Geometry check sheet. Reference: drawing and pictorial views, mm from the part's lowest x, y, z. A direction names the side the tool comes from. Give positions to 0.01 mm unless a question says otherwise; leave off trailing zeros. Order: outer loops, then holes, each group sorted by start corner. A loop starts at its lowest first (then second) coordinate and runs counter-clockwise, first axis right, second up. Notation, with made-up numbers: (20.5, 64) - (74.5, 64) arc R16 ccw to (74.5, 77) - close; hole circle Ø3 at (35.25, 23). An arc over 180 degrees is marked (long way). Answer as a JSON object with one key per item and string values.
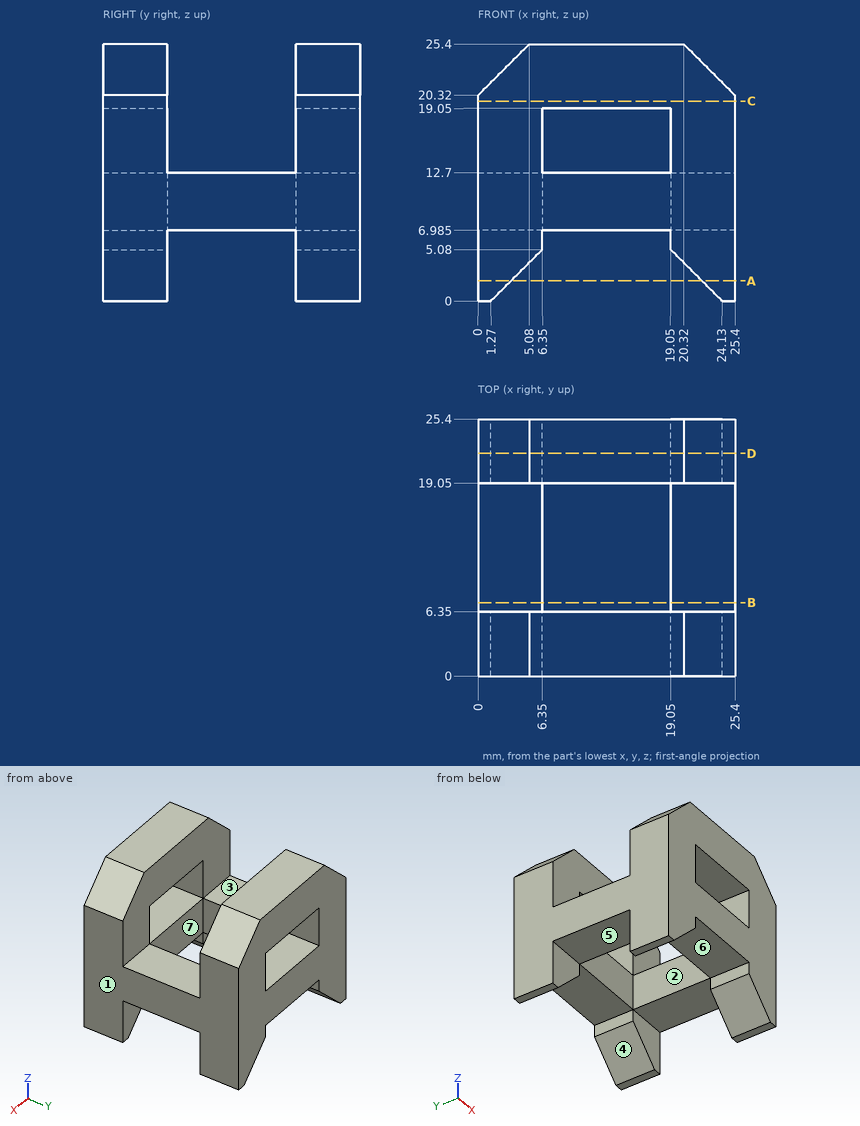
(1) Section check B-B (y = 7.25). Record the cut outline in (x, z) (3 decimals), then the cut area to 3 significant figures.
Computed values:
{"outline": "(0, 6.985) - (6.35, 6.985) - (6.35, 12.7) - (0, 12.7) - close; (19.05, 6.985) - (25.4, 6.985) - (25.4, 12.7) - (19.05, 12.7) - close", "area": "72.6 mm²"}
(2) Material ranges on line 1 along X through (y, z) = (8.5, 10.25); line 2 along X through (y, z) = (24, 4.5), recorded low to high. Write a range as [from, to].
Computed values:
{"line 1": "x = [0, 6.35], [19.05, 25.4]", "line 2": "x = [0, 5.77], [19.63, 25.4]"}
(3) Release check for a two-part mould opening along X. For the marked faces 1, 2, 3 and 4 record: pulls with the +X half, pulls with the -X half, needs draft (parallel to the pull), parting line crosses it, or undercut.
Computed values:
{"face 1": "pulls with the +X half", "face 2": "undercut", "face 3": "needs draft", "face 4": "undercut"}
(4) Section check C-C (z = 19.75). Record the cut outline in (x, y), then the cut area to 3 significant figures.
Computed values:
{"outline": "(0, 0) - (25.4, 0) - (25.4, 6.35) - (0, 6.35) - close; (0, 19.05) - (25.4, 19.05) - (25.4, 25.4) - (0, 25.4) - close", "area": "323 mm²"}
(5) Access from +Z, -Z, +X, -X, +Y, -Y to the whole of each face (thin tool, end or side, straight path). Record for the marked faces 5, 6 and 7.
Computed values:
{"face 5": "-Z, +X, -X", "face 6": "-Z, +Y, -Y", "face 7": "+Z, -Z"}
(6) Section check D-D (y = 22). Record the cut outline in (x, z) (3 decimals).
Computed values:
{"outline": "(0, 0) - (1.27, 0) - (6.35, 5.08) - (6.35, 6.985) - (19.05, 6.985) - (19.05, 5.08) - (24.13, 0) - (25.4, 0) - (25.4, 20.32) - (20.32, 25.4) - (5.08, 25.4) - (0, 20.32) - close; hole (6.35, 12.7) - (19.05, 12.7) - (19.05, 19.05) - (6.35, 19.05) - close"}
(7) Section check A-A (z = 2). Record the cut outline in (x, y), then the cut area to 3 significant figures.
Computed values:
{"outline": "(0, 0) - (3.27, 0) - (3.27, 6.35) - (0, 6.35) - close; (0, 19.05) - (3.27, 19.05) - (3.27, 25.4) - (0, 25.4) - close; (22.13, 0) - (25.4, 0) - (25.4, 6.35) - (22.13, 6.35) - close; (22.13, 19.05) - (25.4, 19.05) - (25.4, 25.4) - (22.13, 25.4) - close", "area": "83.1 mm²"}
(8) Gauge pin test, flat ends, axial feed: pin 1 Ø1.9 at (x, y) = (13.5, 22) entering from -Z (3 decimals); pin 2 Ø3 at (x, y) = (4, 12) entering from +Z. Record the tip position at first contact, or that the pin passes through.
Computed values:
{"pin 1": "stops at z = 6.985", "pin 2": "stops at z = 12.7"}
